Autodesk Inventor part; units mm, degrees
ref_plane "YZ Plane" through (0, 0, 0) normal (1, 0, 0) x (0, 1, 0)
ref_plane "XZ Plane" through (0, 0, 0) normal (0, 1, 0) x (-1, 0, 0)
ref_plane "XY Plane" through (0, 0, 0) normal (0, 0, 1) x (1, 0, 0)
sketch "Sketch1" plane through (0, 0, 0) normal (0, 0, 1) x (1, 0, 0)
  line L0 (0, 2.159) -> (0, -2.159)
  line L1 (0, -2.159) -> (-61.595, -2.159)
  line L2 (0, 2.159) -> (-61.595, 2.159)
  line L3 (-61.595, -38.6842) -> (-14.4526, -38.6842)
  line L4 (-70.231, -13.1699) -> (-70.231, -23.3299)
  line L5 (-74.549, -13.1699) -> (-74.549, -23.3299)
  line L6 (-70.231, -13.1699) -> (-70.231, -2.159)
  line L7 (-70.231, -2.159) -> (-61.595, -2.159)
  line L8 (-61.595, 2.159) -> (-74.549, 2.159)
  line L9 (-74.549, 2.159) -> (-74.549, -13.1699)
  line L10 (-74.549, -23.3299) -> (-74.549, -38.6842)
  line L11 (-74.549, -38.6842) -> (-61.595, -38.6842)
  line L12 (-14.4526, -34.3662) -> (-14.4526, -36.5252)
  line L13 (-14.4526, -36.5252) -> (-14.4526, -38.6842)
  line L14 (-14.4526, -34.3662) -> (-70.231, -34.3662)
  line L15 (-70.231, -34.3662) -> (-70.231, -23.3299)
  point P0 (0, 0)
  point P1 (0, 0)
  point P2 (-61.595, 0)
  point P3 (-72.39, -18.2499)
  point P4 (-72.39, -13.1699)
  point P5 (-72.39, -23.3299)
  dimension "d0" = 61.595
  dimension "d1" = 18.2499
  dimension "d2" = 10.795
  dimension "d3" = 5.08
  dimension "d4" = 5.08
  dimension "d8" = 2.159
  dimension "d9" = 2.159
  dimension "d14" = 2.159
  dimension "d15" = 2.159
  dimension "d34" = 2.159
  dimension "d35" = 47.1424
  dimension "d36" = 36.5252
extrude "Extrusion1" add sketch "Sketch1" along normal blind 4.318
fillet "Fillet10" radius 12.7 2 edges at (-74.549, 2.159, 2.159) (-74.549, -38.6842, 2.159)
fillet "Fillet11" radius 8.382 2 edges at (-70.231, -34.3662, 2.159) (-70.231, -2.159, 2.159)
fillet "Fillet12" radius 2.159 20 edges at (-70.8293, -1.5607, 0) (-74.549, -18.2499, 0) (-70.8293, -34.9645, 0) (-38.0238, -38.6842, 0) (-30.7975, 2.159, 0) (-70.8293, -1.5607, 4.318) (-74.549, -18.2499, 4.318) (-70.8293, -34.9645, 4.318) (-38.0238, -38.6842, 4.318) (-61.722, 2.159, 4.318) (-67.776, -31.9112, 4.318) (-70.231, -18.2499, 4.318) (-67.776, -4.614, 4.318) (-30.7975, -2.159, 4.318) (-38.1508, -34.3662, 4.318) (-67.776, -31.9112, 0) (-70.231, -18.2499, 0) (-67.776, -4.614, 0) (-30.7975, -2.159, 0) (-38.1508, -34.3662, 0)
sketch "Sketch5" plane through (0, 0, 2.159) normal (1, 0, 0) x (0, 0, -1)
  circle A0 centre (0, 0) radius 2.159
  point P0 (2.159, 0)
extrude "Extrusion5" cut sketch "Sketch5" against normal blind 1.27
sketch "Sketch6" plane through (-14.4526, -36.5252, 2.159) normal (1, 0, 0) x (0, 0, -1)
  circle A0 centre (0, 0) radius 2.1591
  point P0 (2.159, 36.5252)
extrude "Extrusion6" cut sketch "Sketch6" against normal blind 0.7874
properties part number "Water_tube" material "Water"
Input: part model. Units: mm. Frame: model coordinates. Round coordinates to 2 decimals unless told otherwise and drop trailing zeros. Write each loop counter-clockwise with the first axis right and the second up, starting at its lowest first coordinate (ties: lowest second). Pieces come first, ordered by that corner, then holes.
1) Ray query, L1, parallel to Y at x = -53, z = 2.35; L2, parallel to Y at x = -57.5, z = 1.1; L3, parallel to X at y = -13.5, z = 1.25. Return the intervals inside material, ascending.
2) Draft query along Y for faces 1 (the cylindrical face through (-38.87, -34.98, 0.65)), 2 (the cylindrical face through (-38.871, -35.015, 3.702)), 3 (the flat face through (-1.27, 0, 2)). Return one class per face: pulls with the +Y half, pulls with the -Y half, needs draft (parallel to the pull), parting line crosses it, or undercut.
3) Contact query for flat-ended pins moving along their axis: P1, Ø2, axis at y = -2.5, z = 0.5, coming from the +X side; P2, Ø2, axis at y = -24, z = 0.5, coming from the +X side; P3, Ø2, axis at y = -13, z = 3, coming from the +X side; P4, Ø2, axis at x = -15, z = 1, coming from the +Y side. Output: stop coordinate, or through.
4) Cut plane C-C (z = 1.3). Return the cut outline in (x, y).
Geometry says:
1. L1: y = -38.68 to -34.37, -2.15 to 2.15
1. L2: y = -38.41 to -34.64, -1.88 to 1.88
1. L3: x = -74.35 to -70.43
2. face 1: undercut
2. face 2: undercut
2. face 3: needs draft
3. P1: stops at x = -1.27
3. P2: stops at x = -70.33
3. P3: stops at x = -70.23
3. P4: stops at y = 2.15
4. outline: (-74.37, -25.98) arc R12.52 ccw to (-61.85, -38.51) - (-15.24, -38.51) - (-15.24, -34.54) - (-61.85, -34.54) arc R8.56 cw to (-70.41, -25.98) - (-70.41, -10.54) arc R8.56 cw to (-61.85, -1.98) - (-1.27, -1.98) - (-1.27, 1.98) - (-61.85, 1.98) arc R12.52 ccw to (-74.37, -10.54) - close
